CAD build for the part. Positions are in the model's coordinates, mm. Coordinates: 2 decimals unless noted, no trailing zeros. Loops run counter-clockwise (first coordinate to the right, second up) from the corner with the lowest first, then second, coordinate; pieces in that order, holes last. Notation, with made-up numbers: (61.5, 64) -> (111.5, 64) arc R31 ccw to (111.5, 89) -> close; hole circle Ø2 at (31.25, -22). An arc over 180 degrees is marked (long way). Answer as a JSON object with one key per item and string values. Group by question number.
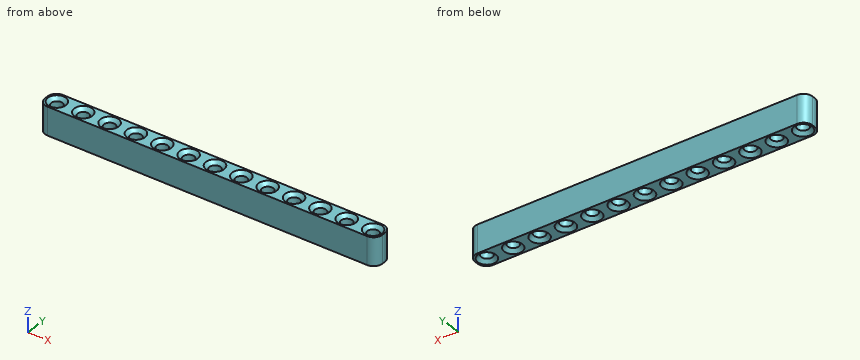
from build123d import *

# Parameters (mm, degrees)
SKETCH1_R           = 1.6
BOSS_EXTRUDE1_DEPTH = 8
CHAMFER1_SIZE       = 1


with BuildPart() as part:
    # Sketch1 → Boss-Extrude1 (new body)
    with BuildSketch(Plane.XY):
        with BuildLine():
            Line((-0.5, 3), (90.5, 3))
            ThreePointArc((90.5, 3), (92.267766953, 2.267766953), (93, 0.5))
            Line((93, 0.5), (93, -0.5))
            ThreePointArc((93, -0.5), (92.267766953, -2.267766953), (90.5, -3))
            Line((90.5, -3), (-0.5, -3))
            ThreePointArc((-0.5, -3), (-2.267766953, -2.267766953), (-3, -0.5))
            Line((-3, -0.5), (-3, 0.5))
            ThreePointArc((-3, 0.5), (-2.267766953, 2.267766953), (-0.5, 3))
        make_face()
        Circle(SKETCH1_R, mode=Mode.SUBTRACT)
        with Locations((7.5, 0)):
            Circle(SKETCH1_R, mode=Mode.SUBTRACT)
        with Locations((15, 0)):
            Circle(SKETCH1_R, mode=Mode.SUBTRACT)
        with Locations((22.5, 0)):
            Circle(SKETCH1_R, mode=Mode.SUBTRACT)
        with Locations((30, 0)):
            Circle(SKETCH1_R, mode=Mode.SUBTRACT)
        with Locations((37.5, 0)):
            Circle(SKETCH1_R, mode=Mode.SUBTRACT)
        with Locations((45, 0)):
            Circle(SKETCH1_R, mode=Mode.SUBTRACT)
        with Locations((52.5, 0)):
            Circle(SKETCH1_R, mode=Mode.SUBTRACT)
        with Locations((60, 0)):
            Circle(SKETCH1_R, mode=Mode.SUBTRACT)
        with Locations((67.5, 0)):
            Circle(SKETCH1_R, mode=Mode.SUBTRACT)
        with Locations((75, 0)):
            Circle(SKETCH1_R, mode=Mode.SUBTRACT)
        with Locations((82.5, 0)):
            Circle(SKETCH1_R, mode=Mode.SUBTRACT)
        with Locations((90, 0)):
            Circle(SKETCH1_R, mode=Mode.SUBTRACT)
    extrude(amount=BOSS_EXTRUDE1_DEPTH)

    # Chamfer1
    chamfer1_edges = [part.edges().sort_by_distance(p)[0] for p in [
        (-1.6, 0, 0),
        (-1.6, 0, 8),
        (5.9, 0, 0),
        (5.9, 0, 8),
        (13.4, 0, 0),
        (13.4, 0, 8),
        (20.9, 0, 0),
        (20.9, 0, 8),
        (28.4, 0, 0),
        (28.4, 0, 8),
        (35.9, 0, 0),
        (35.9, 0, 8),
        (43.4, 0, 0),
        (43.4, 0, 8),
        (50.9, 0, 0),
        (50.9, 0, 8),
        (58.4, 0, 0),
        (58.4, 0, 8),
        (65.9, 0, 0),
        (65.9, 0, 8),
        (73.4, 0, 0),
        (73.4, 0, 8),
        (80.9, 0, 0),
        (80.9, 0, 8),
        (88.4, 0, 0),
        (88.4, 0, 8),
    ]]
    chamfer(chamfer1_edges, length=CHAMFER1_SIZE)


solid = part.part
Item 1: Drill centre lines: L1, parallel to Y at x = 37.5, z = 5.7; L2, parallel to X at y = 1.85, z = 6.5; L3, parallel to Y at x = 9, z = 7.25. Where is each one in solid material? Low to high.
Item 2: Band-saw the part on A-A, the plane z = 5.5. Count the separate pieces of the cut face and the enclosed holes in it, and give its area (3 significant figures).
Item 3: Band-saw the part on B-B, the plane x = 67.5. List the corners of the cut face in (y, z).
Item 4: Flat gauge pins, fed straight in: P1, Ø1.9, axis at x = 22.5, y = 0, coming from the +Z side; P2, Ø3.5, axis at x = 90, y = 0, coming from the +Z side; P3, Ø3.5, axis at x = 15, y = 0, coming from the -Z side. Where does each tip first touch, or does it go through?
Reply:
{
 "1": {"L1": "-3 to -1.6, 1.6 to 3", "L2": "-2.6 to 92.6", "L3": "-3 to -1.08, 1.08 to 3"},
 "2": {"separate pieces": "1", "enclosed holes": "13", "area": "466 mm²"},
 "3": {"outline": "(-3, 0) -> (-2.6, 0) -> (-1.6, 1) -> (-1.6, 7) -> (-2.6, 8) -> (-3, 8) -> close; (1.6, 1) -> (2.6, 0) -> (3, 0) -> (3, 8) -> (2.6, 8) -> (1.6, 7) -> close"},
 "4": {"P1": "through", "P2": "z = 7.15", "P3": "z = 0.85"}
}
